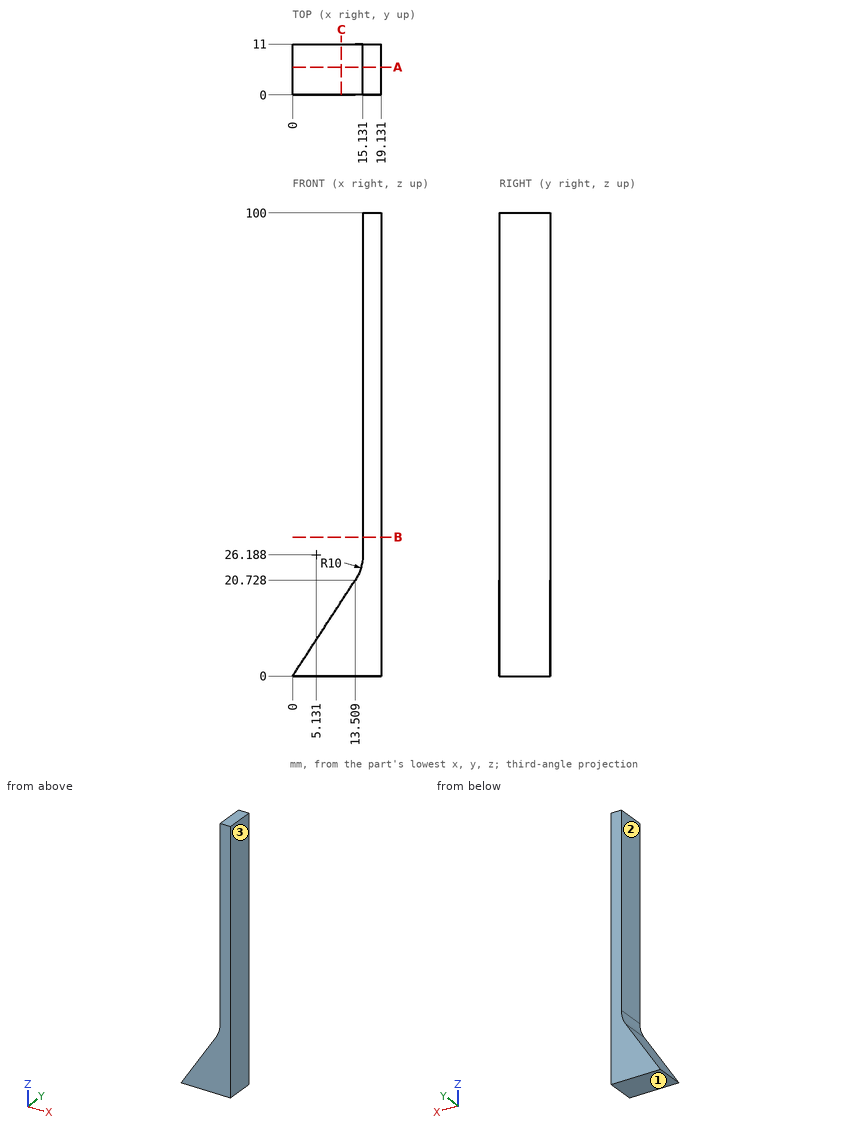
Print and shaded views of the part. All mm, measured from the part's lowest x, y and z. Coordinates: 2 decimals unless noted, no trailing zeros. Order: outer loops, then holes, each group sorted by start corner. A loop starts at its lowest first (then second) coordinate and runs counter-clockwise, first axis right, second up. Notation, with made-up numbers: (21.25, -2) - (66.25, -2) arc R21 cw to (66.25, 4) - close; hole circle Ø8 at (19.25, 81). An arc over 180 degrees is marked (long way). Return JSON: item names as keys, results as strings. Group by question number.
Item 1: Cut at A-A (y = 6). List the corners of the cut face in (x, z).
Item 2: Cut at C-C (x = 10.5). List the corners of the cut face in (y, z).
Item 3: Pin check, flat tips, straight feed: pin 1 (3 mm diameter, centred on x = 7.5, y = 9.5, fed in from +Z); pin 2 (6 mm diameter, centred on y = 2, z = 15.5, fed in from -X) (1 decimal). Stop position of each tip, or through.
Item 4: Cut at B-B (z = 30). List the corners of the cut face in (x, y), plus the area to 3 significant figures.
Item 5: Drill centre lines: probe 1 along X at (y, z) = (4.75, 94); probe 2 along Z at (x, y) = (13.5, 9) (1 decimal); probe 3 along Z at (x, y) = (9.5, 9) (1 decimal). Where is each one in solid material? Low to high. Write a range as from..to.
Item 6: Pull direction X, two halves, no side cores. Call the marked faces 1, 2 and 3: pulls with the +X half, pulls with the -X half, needs draft (parallel to the pull), parting line crosses it, or undercut.
Check values:
{
 "1": {"outline": "(0, 0) - (19.13, 0) - (19.13, 100) - (15.13, 100) - (15.13, 26.19) arc R10 cw to (13.51, 20.73) - close"},
 "2": {"outline": "(0, 0) - (11, 0) - (11, 16.11) - (0, 16.11) - close"},
 "3": {"pin 1": "stops at z = 13.81", "pin 2": "stops at x = 8.1"},
 "4": {"outline": "(15.13, 0) - (19.13, 0) - (19.13, 11) - (15.13, 11) - close", "area": "44.0 mm2"},
 "5": {"probe 1": "x = 15.13..19.13", "probe 2": "z = 0..20.7", "probe 3": "z = 0..14.6"},
 "6": {"face 1": "needs draft", "face 2": "pulls with the -X half", "face 3": "pulls with the +X half"}
}
